Part model, mm, in its own coordinate system. Face numbers are marked on the shaded views. Give positions to 0.01 mm unless a question says otherwise; leave off trailing zeros. Order: outer loops, then holes, each group sorted by start corner. A loop starts at its lowest first (then second) coordinate and runs counter-clockwise, first axis right, second up.
1. Probe line 1 (Z direction, x = -12.5, y = 7.2); line 2 (X direction, y = 3.75, z = -69.1); line 3 (X direction, y = 7.2, z = -7.5). List the from-to ranges inside material, lowest first.
2. Drop flat-ended pins along their axis: pin 1 Ø3 at (x, y) = (-9, 12.5) entering from -Z; pin 2 Ø5 at (x, z) = (15.5, -55.5) entering from +Y; pin 3 Ø6 at (x, z) = (-22.5, -33.5) entering from -Y; pin 4 Ø8 at (x, z) = (15.5, -52.5) entering from +Y. Give the stop position or say it passes through.
3. Mould opens along X. For the marked faces 1 and 2 say: +X half, -X half, draft (parallel to the pull), parting line (faces both ways), or undercut.
4. Slice it at B-B on x = -34.05. Give the number of separate pieces and of enclosed holes in the cut face, and give its area (3 significant figures).
5. Slice it at A-A on y = 8.5. List the corners of the cut face in (x, z).
from build123d import *

# Parameters (mm, degrees)
SKETCH_1_W                   = 75
SKETCH_1_H                   = 92
EXTRUDE_1488_DEPTH           = 7.5
SKETCH_16_W                  = 7.1
SKETCH_16_H                  = 53
CUT_EXTRUDE_2987_DEPTH       = 1
HOLE_WIZARD_M3_D             = 1.6
HOLE_WIZARD_15_M3_AT_2_COUNT = 2
HOLE_WIZARD_15_M3_AT_2_PITCH = 25
HOLE_WIZARD_15_M3_AT_3_COUNT = 2
HOLE_WIZARD_15_M3_AT_3_PITCH = 35.355339059
HOLE_WIZARD_15_M3_AT_4_COUNT = 2
HOLE_WIZARD_15_M3_AT_4_PITCH = 25
SKETCH_28_R                  = 11
CUT_EXTRUDE_6514_DEPTH       = 81.64428064
HOLE_WIZARD_6682_AT_2_COUNT  = 2
HOLE_WIZARD_6682_AT_2_PITCH  = 31
HOLE_WIZARD_6682_AT_3_COUNT  = 2
HOLE_WIZARD_6682_AT_3_PITCH  = 43.840620434
HOLE_WIZARD_6682_AT_4_COUNT  = 2
HOLE_WIZARD_6682_AT_4_PITCH  = 31
SKETCH_90_W                  = 10
SKETCH_90_H                  = 5
EXTRUDE_8536_DEPTH           = 6.5
EXTRUDE_9344_DEPTH           = 2.3
HOLE_WIZARD_M3_2_D           = 2.5
SKETCH_77_W                  = 62
SKETCH_77_H                  = 34
CUT_EXTRUDE_1_DEPTH          = 2
HOLE_WIZARD_M3_3_D           = 2.5
HOLE_WIZARD_M3_3_DEPTH       = 5
HOLE_WIZARD_M3_3_CSINK_D     = 3.05
HOLE_WIZARD_M3_3_CSINK_ANGLE = 90
HOLE_WIZARD_M3_3_TIP         = 0.751075774
HOLE_WIZARD_M3_4_D           = 2.5
HOLE_WIZARD_M3_4_DEPTH       = 5
HOLE_WIZARD_M3_4_TIP         = 0.751075774
HOLE_WIZARD_M3_5_D           = 3.4
HOLE_WIZARD_M3_5_CSINK_D     = 6.3
HOLE_WIZARD_M3_5_CSINK_ANGLE = 90
SKETCH_63_R                  = 1.495
CUT_EXTRUDE_15431_DEPTH      = 81.64428064
FILLET_2_R                   = 1.5
PATTERN_LINEAR_2_COUNT       = 3
PATTERN_LINEAR_2_PITCH       = 15
HOLE_WIZARD_1_M4_D           = 3.3
HOLE_WIZARD_1_M4_DEPTH       = 16
HOLE_WIZARD_1_M4_CSINK_D     = 4.05
HOLE_WIZARD_1_M4_CSINK_ANGLE = 90
HOLE_WIZARD_1_M4_TIP         = 0.991420021
HOLE_WIZARD_2_3_D            = 3.3
HOLE_WIZARD_2_3_DEPTH        = 16
HOLE_WIZARD_2_3_CSINK_D      = 4.05
HOLE_WIZARD_2_3_CSINK_ANGLE  = 90
HOLE_WIZARD_2_3_TIP          = 0.991420021
HOLE_WIZARD_M3_6_D           = 2.5
HOLE_WIZARD_3_D              = 2.5
FILLET_3_R                   = 3


with BuildPart() as part:
    # Эскиз1 → Extrude 1488 (new body)
    with BuildSketch(Plane(origin=(0, 0, 0), x_dir=(1, 0, 0), z_dir=(0, 1, 0))):
        with Locations((0, 25)):
            Rectangle(SKETCH_1_W, SKETCH_1_H)
    extrude(amount=EXTRUDE_1488_DEPTH)

    # Эскиз16 → Cut-Extrude 2987 (cut)
    with BuildSketch(Plane(origin=(0, 7.5, 0), x_dir=(1, 0, 0), z_dir=(0, 1, 0))):
        with Locations((-18, 5.5)):
            Rectangle(SKETCH_16_W, SKETCH_16_H)
        with Locations((18, 5.5)):
            Rectangle(SKETCH_16_W, SKETCH_16_H)
    extrude(amount=-CUT_EXTRUDE_2987_DEPTH, mode=Mode.SUBTRACT)

    # Hole Wizard M3 (through all)
    with Locations(Plane(origin=(0, 6.5, 0), x_dir=(1, 0, 0), z_dir=(0, 1, 0))):
        with Locations((-18, -15), (18, -15)):
            hole_wizard_m3 = Hole(HOLE_WIZARD_M3_D / 2)

    # Эскиз56 → Каретка 15 - M3 (revolve, cut)
    with BuildSketch(Plane(origin=(-12.5, 7.5, -7.5), x_dir=(0, 0, 1), z_dir=(1, 0, 0))):
        Polygon((0, 0), (0, 7.5), (1.7, 7.5), (1.7, 2.45), (3.15, 1), (3.15, 0), align=None)
    hole_wizard_15_m3 = revolve(axis=Axis((-12.5, 13.85, -7.5), (0, -1, 0)), mode=Mode.SUBTRACT)

    # Каретка 15 - M3 at 2: Каретка 15 - M3 ×2
    with Locations(*[(0, 0, i * HOLE_WIZARD_15_M3_AT_2_PITCH) for i in range(1, HOLE_WIZARD_15_M3_AT_2_COUNT)]):
        add(hole_wizard_15_m3, mode=Mode.SUBTRACT)

    # Каретка 15 - M3 at 3: Каретка 15 - M3 ×2
    with Locations(*[Vector(0.7071067811865475, 0, 0.7071067811865476) * (i * HOLE_WIZARD_15_M3_AT_3_PITCH) for i in range(1, HOLE_WIZARD_15_M3_AT_3_COUNT)]):
        add(hole_wizard_15_m3, mode=Mode.SUBTRACT)

    # Каретка 15 - M3 at 4: Каретка 15 - M3 ×2
    with Locations(*[(i * HOLE_WIZARD_15_M3_AT_4_PITCH, 0, 0) for i in range(1, HOLE_WIZARD_15_M3_AT_4_COUNT)]):
        add(hole_wizard_15_m3, mode=Mode.SUBTRACT)

    # Эскиз28 → Cut-Extrude 6514 (cut, through all)
    with BuildSketch(Plane(origin=(0, 7.5, 0), x_dir=(1, 0, 0), z_dir=(0, 1, 0))):
        with Locations(Location((0, 40, 0), (0, 0, 270))):
            Circle(SKETCH_28_R)
    extrude(amount=-CUT_EXTRUDE_6514_DEPTH, mode=Mode.SUBTRACT)

    # Эскиз31 → Hole Wizard 6682 (revolve, cut)
    with BuildSketch(Plane(origin=(-15.5, 7.5, -55.5), x_dir=(0, 0, 1), z_dir=(1, 0, 0))):
        Polygon((0, 0), (0, 7.5), (1.45, 7.5), (1.45, 2.3), (2.75, 1), (2.75, 0), align=None)
    hole_wizard_6682 = revolve(axis=Axis((-15.5, 13.85, -55.5), (0, -1, 0)), mode=Mode.SUBTRACT)

    # Hole Wizard 6682 at 2: Hole Wizard 6682 ×2
    with Locations(*[(i * HOLE_WIZARD_6682_AT_2_PITCH, 0, 0) for i in range(1, HOLE_WIZARD_6682_AT_2_COUNT)]):
        add(hole_wizard_6682, mode=Mode.SUBTRACT)

    # Hole Wizard 6682 at 3: Hole Wizard 6682 ×2
    with Locations(*[Vector(0.7071067811865476, 0, 0.7071067811865476) * (i * HOLE_WIZARD_6682_AT_3_PITCH) for i in range(1, HOLE_WIZARD_6682_AT_3_COUNT)]):
        add(hole_wizard_6682, mode=Mode.SUBTRACT)

    # Hole Wizard 6682 at 4: Hole Wizard 6682 ×2
    with Locations(*[(0, 0, i * HOLE_WIZARD_6682_AT_4_PITCH) for i in range(1, HOLE_WIZARD_6682_AT_4_COUNT)]):
        add(hole_wizard_6682, mode=Mode.SUBTRACT)

    # Эскиз90 → Extrude 8536 (add)
    with BuildSketch(Plane(origin=(0, 7.5, 0), x_dir=(1, 0, 0), z_dir=(0, 1, 0))):
        with Locations((18, 34.5)):
            Rectangle(SKETCH_90_W, SKETCH_90_H)
        with Locations((-18, 34.5)):
            Rectangle(SKETCH_90_W, SKETCH_90_H)
    extrude(amount=EXTRUDE_8536_DEPTH)

    # Эскиз87 → Extrude 9344 (add)
    with BuildSketch(Plane(origin=(0, 7.5, 0), x_dir=(1, 0, 0), z_dir=(0, 1, 0))):
        with BuildLine():
            Line((-6, 57), (6, 57))
            ThreePointArc((6, 57), (9, 54), (6, 51))
            Line((6, 51), (-6, 51))
            ThreePointArc((-6, 51), (-9, 54), (-6, 57))
        make_face()
    extrude(amount=EXTRUDE_9344_DEPTH)

    # Hole Wizard M3 2 (through all)
    with Locations(Plane(origin=(0, 9.8, 0), x_dir=(-1, 0, 0), z_dir=(0, 1, 0))):
        with Locations((6, -54), (-6, -54)):
            Hole(HOLE_WIZARD_M3_2_D / 2)

    # Эскиз77 → Вырез-Вытянуть1 (cut)
    with BuildSketch(Plane.XZ):
        with Locations((0, 5)):
            Rectangle(SKETCH_77_W, SKETCH_77_H)
    extrude(amount=-CUT_EXTRUDE_1_DEPTH, mode=Mode.SUBTRACT)

    # Hole Wizard M3 3
    with Locations(Plane(origin=(0, 0, -71), x_dir=(-1, 0, 0), z_dir=(0, 0, -1))):
        with Locations((-30, 3.75), (0, 3.75), (30, 3.75)):
            CounterSinkHole(HOLE_WIZARD_M3_3_D / 2, HOLE_WIZARD_M3_3_CSINK_D / 2, depth=HOLE_WIZARD_M3_3_DEPTH, counter_sink_angle=HOLE_WIZARD_M3_3_CSINK_ANGLE)
            with Locations((0, 0, -(HOLE_WIZARD_M3_3_DEPTH + HOLE_WIZARD_M3_3_TIP / 2))):  # 118° drill point
                Cone(0, HOLE_WIZARD_M3_3_D / 2, HOLE_WIZARD_M3_3_TIP, mode=Mode.SUBTRACT)

    # Hole Wizard M3 4
    with Locations(Plane.XY.offset(21)):
        with Locations((-30, 3.75), (0, 3.75), (30, 3.75)):
            Hole(HOLE_WIZARD_M3_4_D / 2, depth=HOLE_WIZARD_M3_4_DEPTH)
            with Locations((0, 0, -(HOLE_WIZARD_M3_4_DEPTH + HOLE_WIZARD_M3_4_TIP / 2))):  # 118° drill point
                Cone(0, HOLE_WIZARD_M3_4_D / 2, HOLE_WIZARD_M3_4_TIP, mode=Mode.SUBTRACT)

    # Hole Wizard M3 5 (through all)
    with Locations(Plane(origin=(0, 0, 0), x_dir=(-1, 0, 0), z_dir=(0, -1, 0))):
        with Locations((34.5, 25), (34.5, -16), (34.5, 66), (-34.5, 66), (-34.5, 25), (-34.5, -16)):
            CounterSinkHole(HOLE_WIZARD_M3_5_D / 2, HOLE_WIZARD_M3_5_CSINK_D / 2, counter_sink_angle=HOLE_WIZARD_M3_5_CSINK_ANGLE)

    # Эскиз63 → Cut-Extrude 15431 (cut, through all)
    with BuildSketch(Plane(origin=(0, 7.5, 0), x_dir=(1, 0, 0), z_dir=(0, 1, 0))):
        with Locations(Location((-18, 66, 0), (0, 0, 270))):
            Circle(SKETCH_63_R)
        with Locations(Location((18, 66, 0), (0, 0, 270))):
            Circle(SKETCH_63_R)
    extrude(amount=-CUT_EXTRUDE_15431_DEPTH, mode=Mode.SUBTRACT)

    # Скругление2
    fillet_2_edges = [part.edges().sort_by_distance(p)[0] for p in [
        (-21.55, 7, -32),
        (-14.45, 7, -32),
        (-31, 1, -12),
        (31, 1, -12),
        (21.55, 7, -32),
        (14.45, 7, -32),
    ]]
    fillet(fillet_2_edges, radius=FILLET_2_R)

    # Линейный массив2: Hole Wizard M3 ×3
    with Locations(*[(0, 0, -i * PATTERN_LINEAR_2_PITCH) for i in range(1, PATTERN_LINEAR_2_COUNT)]):
        add(hole_wizard_m3, mode=Mode.SUBTRACT)

    # Трос1-M4
    with Locations(Plane.ZY.offset(37.5)):
        with Locations((0.4, 3.75), (9.6, 3.75)):
            CounterSinkHole(HOLE_WIZARD_1_M4_D / 2, HOLE_WIZARD_1_M4_CSINK_D / 2, depth=HOLE_WIZARD_1_M4_DEPTH, counter_sink_angle=HOLE_WIZARD_1_M4_CSINK_ANGLE)
            with Locations((0, 0, -(HOLE_WIZARD_1_M4_DEPTH + HOLE_WIZARD_1_M4_TIP / 2))):  # 118° drill point
                Cone(0, HOLE_WIZARD_1_M4_D / 2, HOLE_WIZARD_1_M4_TIP, mode=Mode.SUBTRACT)

    # Трос2-М3
    with Locations(Plane(origin=(37.5, 0, 0), x_dir=(0, 0, -1), z_dir=(1, 0, 0))):
        with Locations((-0.4, 3.75), (-9.6, 3.75)):
            CounterSinkHole(HOLE_WIZARD_2_3_D / 2, HOLE_WIZARD_2_3_CSINK_D / 2, depth=HOLE_WIZARD_2_3_DEPTH, counter_sink_angle=HOLE_WIZARD_2_3_CSINK_ANGLE)
            with Locations((0, 0, -(HOLE_WIZARD_2_3_DEPTH + HOLE_WIZARD_2_3_TIP / 2))):  # 118° drill point
                Cone(0, HOLE_WIZARD_2_3_D / 2, HOLE_WIZARD_2_3_TIP, mode=Mode.SUBTRACT)

    # Hole Wizard M3 6 (through all)
    with Locations(Plane(origin=(0, 0, 0), x_dir=(-1, 0, 0), z_dir=(0, -1, 0))):
        with Locations((34.05, 45), (22.95, 45), (-34.05, 45), (-22.95, 45)):
            Hole(HOLE_WIZARD_M3_6_D / 2)

    # Пружина-М3 (through all)
    with Locations(Plane(origin=(0, 7.5, 0), x_dir=(1, 0, 0), z_dir=(0, 1, 0))):
        with Locations((-27.5, 65), (27.5, 65)):
            Hole(HOLE_WIZARD_3_D / 2)

    # Скругление3
    fillet_3_edges = [part.edges().sort_by_distance(p)[0] for p in [
        (23, 10.75, -37),
        (13, 10.75, -37),
        (-23, 10.75, -37),
        (-13, 10.75, -37),
    ]]
    fillet(fillet_3_edges, radius=FILLET_3_R)


solid = part.part
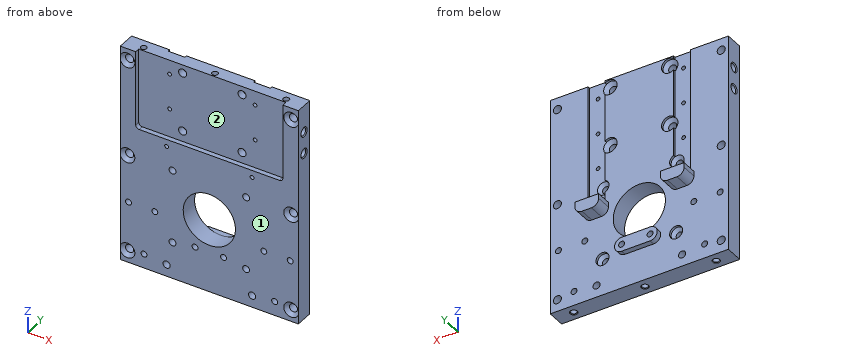
Data:
1. line 1: z = -71 to -10.65, -4.35 to 14.35, 20.65 to 21
1. line 2: x = -37.5 to -31.25, -28.75 to -1.25, 1.25 to 28.75, 31.25 to 37.5
1. line 3: x = -37.5 to -21.55, -9.35 to 9.35, 21.55 to 37.5
2. pin 1: passes through
2. pin 2: stops at y = 6.25
2. pin 3: stops at y = 0
2. pin 4: stops at y = 7.5
3. face 1: draft
3. face 2: undercut
4. separate pieces: 5
4. enclosed holes: 2
4. area: 574 mm2
5. outline: (-23, -34) arc R3 ccw to (-20, -37) - (-16, -37) arc R3 ccw to (-13, -34) - (-13, -32) - (-23, -32) - close; (-6, -57) - (6, -57) arc R3 ccw to (6, -51) - (-6, -51) arc R3 ccw to start; (13, -34) arc R3 ccw to (16, -37) - (20, -37) arc R3 ccw to (23, -34) - (23, -32) - (13, -32) - close; hole circle Ø2.5 at (-6, -54); hole circle Ø2.5 at (6, -54)
